Input: part model. Units: mm. Frame: model coordinates. A direction names the side the tool comes from. Coordinates: 2 decimals unless noted, no trailing zeros. Loops run counter-clockwise (first coordinate to the right, second up) from the corner with the lowest first, then second, coordinate; pieces in that order, holes last. Notation, with made-up numbers: (77, -29) - (96, -29) arc R22 cw to (96, -14) - close; hole circle Ø4 at (49, 78.25). An arc over 180 degrees is marked (long way). Write item = value, one per line. Start each with the question number.
Autodesk Inventor part; units mm, degrees
ref_plane "YZ Plane" through (0, 0, 0) normal (1, 0, 0) x (0, 1, 0)
ref_plane "XZ Plane" through (0, 0, 0) normal (0, 1, 0) x (-1, 0, 0)
ref_plane "XY Plane" through (0, 0, 0) normal (0, 0, 1) x (1, 0, 0)
sketch "Sketch1" plane through (0, 0, 0) normal (0, 1, 0) x (-1, 0, 0)
  line L0 (-550, 230) -> (550, 230)
  line L1 (550, 230) -> (550, -230)
  line L2 (550, -230) -> (-550, -230)
  line L3 (-550, -230) -> (-550, 230)
  line L4 (-550, 230) -> (550, -230) construction
  line L5 (550, 230) -> (-550, -230) construction
  point P0 (0, 0)
  dimension "d0" = 1100
  dimension "d1" = 460
extrude "Extrusion1" add sketch "Sketch1" along normal blind 30
sketch "Sketch2" plane through (0, 30, 0) normal (0, 1, 0) x (1, 0, 0)
  line L0 (-550, 230) -> (-550, -230)
  line L1 (-550, -230) -> (-520, -230)
  line L2 (-520, -230) -> (-520, -200)
  line L3 (-520, -200) -> (-550, -200)
  line L4 (-550, -200) -> (-550, -230)
  line L5 (-550, 230) -> (-520, 230)
  line L6 (-520, 230) -> (-520, 200)
  line L7 (-520, 200) -> (-550, 200)
  line L8 (-550, 200) -> (-550, 230)
  line L9 (550, -230) -> (550, 230)
  line L10 (550, -230) -> (520, -230)
  line L11 (520, -230) -> (520, -200)
  line L12 (520, -200) -> (550, -200)
  line L13 (550, -200) -> (550, -230)
  line L14 (550, 230) -> (520, 230)
  line L15 (520, 230) -> (520, 200)
  line L16 (520, 200) -> (550, 200)
  line L17 (550, 200) -> (550, 230)
  point P0 (0, 0)
  dimension "d6" = 30
  dimension "d7" = 30
extrude "Extrusion2" cut sketch "Sketch2" against normal blind 30
sketch "Sketch3" plane through (0, 0, 0) normal (0, -1, 0) x (1, 0, 0)
  line L0 (-325, -150) -> (325, -150)
  line L1 (325, -150) -> (325, 150)
  line L2 (325, 150) -> (-325, 150)
  line L3 (-325, 150) -> (-325, -150)
  line L4 (-325, -150) -> (325, 150) construction
  line L5 (325, -150) -> (-325, 150) construction
  point P0 (0, 0)
  dimension "d10" = 650
  dimension "d11" = 300
extrude "Extrusion3" add sketch "Sketch3" along normal blind 30
properties part number "Platform_Arm"
Item 1: Ray query, line 1 (Z direction, x = -258.5, y = -16); line 2 (Y direction, x = 481, z = -69.5); line 3 (X direction, y = -6, z = -2). Return the intervals inside material, ascending.
Item 2: Cut plane A-A on z = 65.5. Return loops of the section in (x, y).
Item 3: Pin query (flat end, axial travel): pin 1 (15 mm diameter, centred on x = 58, y = -14.5, fed in from -Z); pin 2 (1 mm diameter, centred on y = -6, z = 25.5, fed in from -X); pin 3 (15 mm diameter, centred on x = 539, y = 15, fed in from +Z). Return the tip coordinate at first contact, or that it passes through.
Item 4: Access query for faces 1 (the flat face through (-535, 15, -200)), 2 (the flat face through (-520, 15, 215)), 3 (the flat face through (5, -15, 150)). Directions: +Z, -Z, +X, -X, +Y, -Y. A direction counts if a zero-diameter tool reaches every point of the face in a straight line with its end or side. Return the directions, or none.
Item 5: Cut plane D-D on x = -377.5. Return loops of the section in (y, z), plus the area to 3 significant figures.
Item 6: Cut plane C-C on y = -11.5. Return loops of the section in (x, z).
Item 7: Cut plane B-B on x = -130.5. Return loops of the section in (y, z).
Recorded:
q1.line_1 = -150 to 150
q1.line_2 = 0 to 30
q1.line_3 = -325 to 325
q2.outline = (-550, 0) - (-325, 0) - (-325, -30) - (325, -30) - (325, 0) - (550, 0) - (550, 30) - (-550, 30) - close
q3.pin_1 = -150
q3.pin_2 = -325
q3.pin_3 = 200
q4.face_1 = -Z, -X, +Y, -Y
q4.face_2 = +Z, -X, +Y, -Y
q4.face_3 = +Z, +X, -X, -Y
q5.outline = (0, -230) - (30, -230) - (30, 230) - (0, 230) - close
q5.area = 13,800 mm²
q6.outline = (-325, -150) - (325, -150) - (325, 150) - (-325, 150) - close
q7.outline = (-30, -150) - (0, -150) - (0, -230) - (30, -230) - (30, 230) - (0, 230) - (0, 150) - (-30, 150) - close
